from build123d import *

# Parameters (mm, degrees)
F0_W     = 60
F0_H     = 25
F1_DEPTH = 2
F3_DEPTH = 0.6


with BuildPart() as f1:
    # F0 (on Top) → F1 (new body)
    with BuildSketch(Plane.XY):
        Rectangle(F0_W, F0_H)
        with BuildLine():
            ThreePointArc((-16.65, 3.725), (-16.474264, 4.149264), (-16.05, 4.325))
            Line((-16.05, 4.325), (-8.6, 4.325))
            ThreePointArc((-8.6, 4.325), (-8.175736, 4.149264), (-8, 3.725))
            Line((-8, 3.725), (-8, -3.725))
            ThreePointArc((-8, -3.725), (-8.175736, -4.149264), (-8.6, -4.325))
            Line((-8.6, -4.325), (-16.05, -4.325))
            ThreePointArc((-16.05, -4.325), (-16.474264, -4.149264), (-16.65, -3.725))
            Line((-16.65, -3.725), (-16.65, 3.725))
        make_face(mode=Mode.SUBTRACT)
        with BuildLine():
            ThreePointArc((8, 3.725), (8.175736, 4.149264), (8.6, 4.325))
            Line((8.6, 4.325), (16.05, 4.325))
            ThreePointArc((16.05, 4.325), (16.474264, 4.149264), (16.65, 3.725))
            Line((16.65, 3.725), (16.65, -3.725))
            ThreePointArc((16.65, -3.725), (16.474264, -4.149264), (16.05, -4.325))
            Line((16.05, -4.325), (8.6, -4.325))
            ThreePointArc((8.6, -4.325), (8.175736, -4.149264), (8, -3.725))
            Line((8, -3.725), (8, 3.725))
        make_face(mode=Mode.SUBTRACT)
    extrude(amount=F1_DEPTH)

    # F2 (on face) → F3 (cut)
    with BuildSketch(Plane.XY.offset(2)):
        with BuildLine():
            Line((15.225, 8.25), (9.425, 8.25))
            ThreePointArc((9.425, 8.25), (9.000736, 8.074264), (8.825, 7.65))
            Line((8.825, 7.65), (8.825, 4.325))
            Line((8.825, 4.325), (15.825, 4.325))
            Line((15.825, 4.325), (15.825, 7.65))
            ThreePointArc((15.825, 7.65), (15.649264, 8.074264), (15.225, 8.25))
        make_face()
        with BuildLine():
            Line((15.825, -4.325), (8.825, -4.325))
            Line((8.825, -4.325), (8.825, -7.65))
            ThreePointArc((8.825, -7.65), (9.000736, -8.074264), (9.425, -8.25))
            Line((9.425, -8.25), (15.225, -8.25))
            ThreePointArc((15.225, -8.25), (15.649264, -8.074264), (15.825, -7.65))
            Line((15.825, -7.65), (15.825, -4.325))
        make_face()
    extrude(amount=-F3_DEPTH, mode=Mode.SUBTRACT)


solid = f1.part
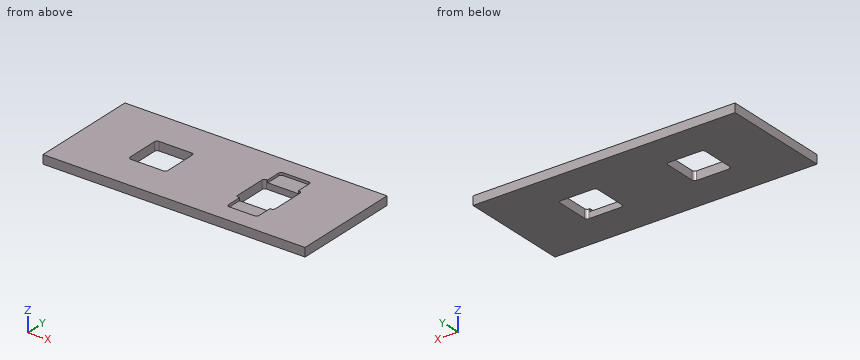
Input: part model. Units: mm. Frame: model coordinates. Give positions to 0.01 mm unless a question says otherwise; leave off trailing zeros. Order: outer loops, then holes, each group sorted by start corner. A loop starts at its lowest first (then second) coordinate and runs counter-clockwise, first axis right, second up.
Q1. Contact query for a flat-ended pin moving along its axis: pin 1 Ø3 at (x, y) = (10.5, 6.5) entering from +Z. Output: stop coordinate, or through.
Checked values:
pin 1: stops at z = 1.4
Q2. Section D-D on y = 5. Output: boundary loops of the cut face in (x, z) (3 decimals).
Checked values:
outline: (-30, 0) - (30, 0) - (30, 2) - (15.825, 2) - (15.825, 1.4) - (8.825, 1.4) - (8.825, 2) - (-30, 2) - close
Q3. Ray query, probe 1 along X at (y, z) = (-1.5, 1.9); probe 2 along X at (y, z) = (-5.5, 1.9) (3 decimals); probe 3 along Y at (x, z) = (11, 1.8). Return the intervals inside material, ascending.
Checked values:
probe 1: x = -30 to -16.65, -8 to 8, 16.65 to 30
probe 2: x = -30 to 8.825, 15.825 to 30
probe 3: y = -12.5 to -8.25, 8.25 to 12.5
Q4. Section C-C on z = 0.8. Output: boundary loops of the cut face in (x, y) (3 decimals), and give its area (3 significant figures).
Checked values:
outline: (-30, -12.5) - (30, -12.5) - (30, 12.5) - (-30, 12.5) - close; hole (-16.65, -3.725) arc R0.6 ccw to (-16.05, -4.325) - (-8.6, -4.325) arc R0.6 ccw to (-8, -3.725) - (-8, 3.725) arc R0.6 ccw to (-8.6, 4.325) - (-16.05, 4.325) arc R0.6 ccw to (-16.65, 3.725) - close; hole (8, -3.725) arc R0.6 ccw to (8.6, -4.325) - (16.05, -4.325) arc R0.6 ccw to (16.65, -3.725) - (16.65, 3.725) arc R0.6 ccw to (16.05, 4.325) - (8.6, 4.325) arc R0.6 ccw to (8, 3.725) - close
area: 1,350 mm2
Q5. Section B-B on y = 1. Output: boundary loops of the cut face in (x, z), and give its area (3 significant figures).
Checked values:
outline: (-30, 0) - (-16.65, 0) - (-16.65, 2) - (-30, 2) - close; (-8, 0) - (8, 0) - (8, 2) - (-8, 2) - close; (16.65, 0) - (30, 0) - (30, 2) - (16.65, 2) - close
area: 85.4 mm2
Q6. Section A-A on x = -15. Output: boundary loops of the cut face in (y, z) (3 decimals).
Checked values:
outline: (-12.5, 0) - (-4.325, 0) - (-4.325, 2) - (-12.5, 2) - close; (4.325, 0) - (12.5, 0) - (12.5, 2) - (4.325, 2) - close
